Drawing for the job (mm, zero at the part's lowest x, y, z). A direction names the side the tool comes from. Coordinates: 2 decimals unless noted, no trailing zeros. Write each loop counter-clockwise with the first axis right and the second up, starting at its lowest first coordinate (ties: lowest second). Pieces come first, ordered by that corner, then holes. Notation, with made-up numbers: (5.5, 7.25) -> (11.5, 7.25) arc R21 cw to (11.5, 35.25) -> close; hole circle Ø3 at (77, -16.75). An arc over 180 degrees is marked (long way). Write item = value, one per line. Start each with the question number.
Q1. Tool access for the marked faces 1 and 2: list every direction of +Z, -Z, +X, -X, +Y, -Y with a clear straight run to the whole face (end or side of a thin tool).
Q2. Band-saw the part on C-C, the plane y = 22. List the corners of the cut face in (x, z), plus the area to 3 significant figures.
Q3. Pull direction Y, two halves, no side cores. Call the marked faces 3, 4 and 5: released by +Y, released by -Y, zero draft, split by the parting line, or undercut.
Q4. Probe line 1 (X direction, y = 19, z = 4.5) (1 decimal); line 2 (X direction, y = 28.85, z = 15); line 3 (X direction, y = 17, z = 15.75) (1 decimal). List the from-to ranges inside material, lowest first.
Q5. Band-saw the part on B-B, the plane x = 77.15. List the corners of the cut face in (y, z), plus the area to 3 significant figures.
Q6. Band-saw the part on D-D, the plane z = 5. List the corners of the cut face in (x, y), plus the area to 3 significant figures.
Q7. Band-saw the part on A-A, the plane z = 15. List the corners of the cut face in (x, y).
Q8. Pin check, flat tips, straight feed: P1, Ø1, axis at y = 8.5, z = 14.5, coming from the -X side; P2, Ø5, axis at x = 32.85, z = 15, coming from the -Y side; P3, Ø8, axis at x = 70.5, y = 21.5, coming from the -Z side; P4, Ø1, axis at y = 9, z = 22, coming from the -X side (1 decimal). Stop position of each tip, or through.
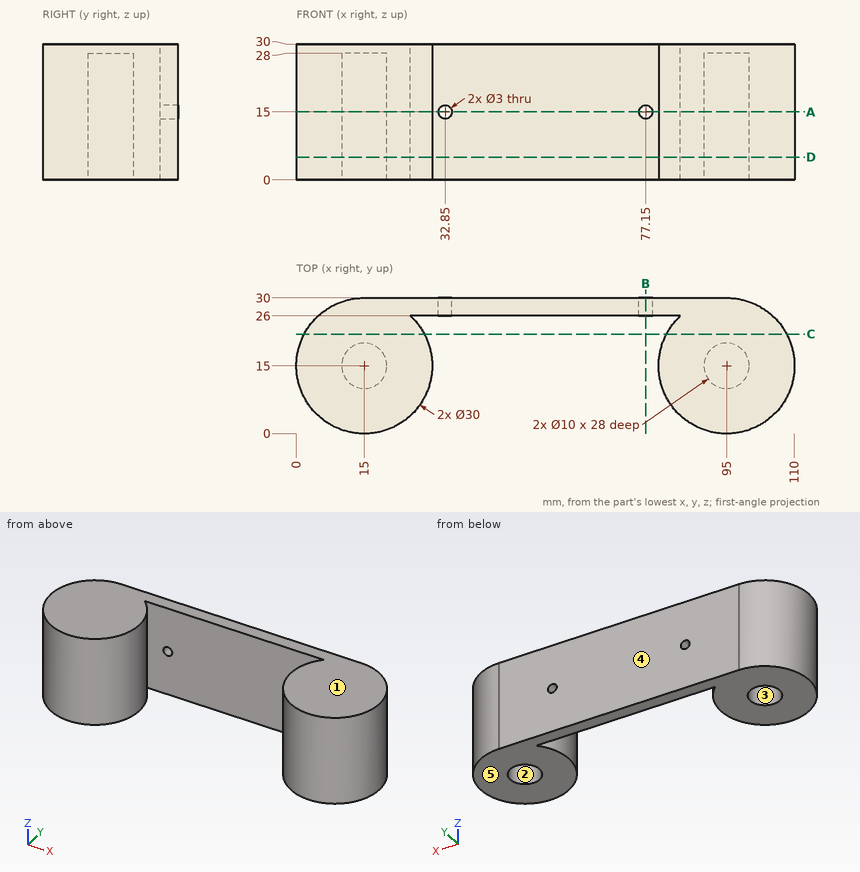
Ans:
q1.face_1 = +Z, +X, -X, +Y, -Y
q1.face_2 = -Z
q2.outline = (1.73, 0) -> (28.27, 0) -> (28.27, 30) -> (1.73, 30) -> close; (81.73, 0) -> (108.27, 0) -> (108.27, 30) -> (81.73, 30) -> close
q2.area = 1,590 mm2
q3.face_3 = undercut
q3.face_4 = released by +Y
q3.face_5 = zero draft
q4.line_1 = 0.5 to 12, 18 to 29.5, 80.5 to 92, 98 to 109.5
q4.line_2 = 9.24 to 31.35, 34.35 to 75.65, 78.65 to 100.76
q4.line_3 = 0.1 to 10.4, 19.6 to 29.9, 80.1 to 90.4, 99.6 to 109.9
q5.outline = (26, 0) -> (30, 0) -> (30, 13.5) -> (26, 13.5) -> close; (26, 16.5) -> (30, 16.5) -> (30, 30) -> (26, 30) -> close
q5.area = 108 mm2
q6.outline = (15, 30) arc R15 ccw (long way) to (25.2, 26) -> (84.8, 26) arc R15 ccw (long way) to (95, 30) -> close; hole circle Ø10 at (15, 15); hole circle Ø10 at (95, 15)
q6.area = 1,520 mm2
q7.outline = (15, 30) arc R15 ccw (long way) to (25.2, 26) -> (31.35, 26) -> (31.35, 30) -> close; (34.35, 26) -> (75.65, 26) -> (75.65, 30) -> (34.35, 30) -> close; (78.65, 26) -> (84.8, 26) arc R15 ccw (long way) to (95, 30) -> (78.65, 30) -> close; hole circle Ø10 at (15, 15); hole circle Ø10 at (95, 15)
q8.P1 = 1.25
q8.P2 = 26
q8.P3 = through
q8.P4 = 1
